Check sheet for the modelled part. Datum: model origin and axes. Units: mm. A direction names the side the tool comes from. Round coordinates to 2 decimals unless told otherwise and drop trailing zeros. Write each loop counter-clockwise with the first axis right and the second up, starting at its lowest first coordinate (ties: lowest second). Pieces come first, ordered by that corner, then holes. Notation, with made-up numbers: M 84,45 L 101,45 A16 cw 101,74 Z; hole C 39.25,21.25 d6. An arc over 180 degrees is marked long. Put each result on its own line as item: value.
```python
from build123d import *

# Parameters (mm, degrees)
F0_W     = 30
F0_H     = 30
F0_R     = 2.75
F1_DEPTH = 5
F2_W     = 30
F2_H     = 30
F3_DEPTH = 5
F4_R     = 6.25
F5_DEPTH = 6
F6_R     = 14.99999
F7_SIZE  = 3


# Not quite as in the source:
# - a fillet or chamfer is up to 0.001 mm smaller than in the source, because OpenCascade refuses the exact size


with BuildPart() as f1:
    # F0 (on Top) → F1 (new body)
    with BuildSketch(Plane.XY):
        with Locations((15, -1.7180653661)):
            Rectangle(F0_W, F0_H)
        with Locations((15, -1.7180653661)):
            Circle(F0_R, mode=Mode.SUBTRACT)
    extrude(amount=F1_DEPTH)

    # F2 (on face) → F3 (join)
    with BuildSketch(Plane(origin=(0, 13.2819346339, 0), x_dir=(-1, 0, 0), z_dir=(0, 1, 0))):
        with Locations((-15, 15)):
            Rectangle(F2_W, F2_H)
    extrude(amount=-F3_DEPTH)

    # F4 (on face) → F5 (cut)
    with BuildSketch(Plane(origin=(0, 13.2819346339, 0), x_dir=(-1, 0, 0), z_dir=(0, 1, 0))):
        with Locations((-15, 19)):
            Circle(F4_R)
    extrude(amount=-F5_DEPTH, mode=Mode.SUBTRACT)

    # F6 (radius 15 in the source; OpenCascade refuses exactly that, so slightly less here)
    f6_edges = [f1.edges().sort_by_distance(p)[0] for p in [
        (30, 10.781935, 30),
        (0, 10.781935, 30),
    ]]
    fillet(f6_edges, radius=F6_R)

    # F7
    f7_edges = [f1.edges().sort_by_distance(p)[0] for p in [
        (12.25, -1.718065, 5),
    ]]
    chamfer(f7_edges, length=F7_SIZE)


solid = f1.part
```
1. Scan lines: probe 1 along Y at (x, z) = (15, 0.75); probe 2 along Y at (x, z) = (8.5, 10); probe 3 along Z at (x, y) = (3, 8.25). Record each from-to range of solid material in increasing order.
Computed values:
probe 1: y = -16.72 to -4.47, 1.03 to 13.28
probe 2: y = 8.28 to 13.28
probe 3: z = 0 to 5
2. Cross-section at D-D (z = 26.5). Enter the section's corners in (x, y).
Computed values:
outline: M 5.37,8.28 L 24.63,8.28 L 24.63,13.28 L 5.37,13.28 Z
3. Depth check by flat-ended pin: pin 1 Ø12 at (x, z) = (16, 17.5) entering from +Y; pin 2 Ø7.5 at (x, z) = (18.5, 12.5) entering from -Y; pin 3 Ø10 at (x, y) = (3, -13.5) entering from +Z; pin 4 Ø11 at (x, z) = (15, 19) entering from +Y. Enter the tip coordinate at first touch or a pass-through.
Computed values:
pin 1: stops at y = 13.28
pin 2: stops at y = 8.28
pin 3: stops at z = 5
pin 4: passes through
4. Cross-section at C-C (y = -13). Enter the section's corners in (x, z).
Computed values:
outline: M 0,0 L 30,0 L 30,5 L 0,5 Z
5. Cross-section at B-B (x = 2.5). Enter the section's corners in (y, z).
Computed values:
outline: M -16.72,0 L 13.28,0 L 13.28,23.29 L 8.28,23.29 L 8.28,5 L -16.72,5 Z
6. Release check for a two-part mould opening along X. For faces 1 (the flat face through (15, 8.282, 12)), 2 (the cylindrical face through (12.253, -1.597, 0.986)), 3 (the conical face through (12.107, -1.591, 2.146)), 4 (the flat face through (30, 1, 4)) record: +X half, -X half, draft (parallel to the pull), parting line (faces both ways), or undercut.
Computed values:
face 1: draft
face 2: undercut
face 3: undercut
face 4: +X half
7. Cross-section at A-A (z = 17). Enter the section's corners in (x, y).
Computed values:
outline: M 0.13,8.28 L 9.08,8.28 L 9.08,13.28 L 0.13,13.28 Z; M 20.92,8.28 L 29.87,8.28 L 29.87,13.28 L 20.92,13.28 Z
8. Access from +Z, -Z, +X, -X, +Y, -Y to the whole of each face (thin tool, end or side, straight path). Record for faces 5 (the flat face through (11, -7, 5)), 6 (the flat face through (0, 1, 4)).
Computed values:
face 5: +Z, +X, -X, -Y
face 6: +Z, -Z, -X, +Y, -Y
